Design review of the part built by this model. Coordinates are the model's own, in mm. A direction names the side the tool comes from. Give positions to 0.01 mm unless a question says otherwise; leave off trailing zeros. Write each loop counter-clockwise with the first axis right and the second up, starting at its lowest first coordinate (ties: lowest second). Pieces come first, ordered by that corner, then holes.
```python
from build123d import *

# Parameters (mm, degrees)
F0_W      = 38.1
F0_H      = 19.05
F1_DEPTH  = 50.8
F2_W      = 25.4
F2_H      = 19.05
F3_DEPTH  = 12.7
F5_DEPTH  = 31.75
F8_DEPTH  = 25.4
F10_DEPTH = 107.95
F11_W     = 38.1
F11_H     = 10.8646959405
F12_DEPTH = 50.8
F14_DEPTH = 25.4
F16_DEPTH = 25.4
F17_W     = 12.7
F17_H     = 10.8646959405
F18_DEPTH = 25.4
F6_W      = 2.6920993537
F6_H      = 9.7637060691
F19_DEPTH = 25.4
F20_DEPTH = 25.4
F21_W     = 11.8566676974
F21_H     = 11.0813332722
F22_DEPTH = 6.35
F23_W     = 4.0861964226
F23_H     = 3.3253813162
F23_W_2   = 3.8762353361
F23_H_2   = 3.7055220455
F23_W_3   = 3.8942359388
F23_H_3   = 4.0504299104
F24_DEPTH = 6.35
F26_DEPTH = 38.1
F28_DEPTH = 38.1
F30_DEPTH = 25.4


with BuildPart() as f1:
    # F0 (on Right) → F1 (new body)
    with BuildSketch(Plane.YZ):
        with Locations((42.7892319858, 20.3896959405)):
            Rectangle(F0_W, F0_H)
        Polygon((23.7392319858, 29.9146959405), (61.8392319858, 29.9146959405), (42.9846160114, 42.6146959405), align=None)
    extrude(amount=F1_DEPTH)

    # F2 (on face) → F3 (join)
    with BuildSketch(Plane.XZ.offset(-23.7392319858)):
        with Locations((25.4, 20.3896959405)):
            Rectangle(F2_W, F2_H)
    extrude(amount=F3_DEPTH)

    # F4 (on face) → F5 (join)
    with BuildSketch(Plane.XZ.offset(-11.0392319858)):
        Polygon((25.4, 44.1137275976), (12.7, 29.9146959405), (38.1, 29.9146959405), align=None)
    extrude(amount=-F5_DEPTH)

    # F7 (on Top) → F8 (join)
    with BuildSketch(Plane.XY):
        Polygon((0, 23.8369237632), (0, 62.1323101223), (-40.3469242156, 62.1323101223), (-40.3469242156, -46.306155622), (0, -46.306155622), align=None)
    extrude(amount=F8_DEPTH)

    # F9 (on face) → F10 (join)
    with BuildSketch(Plane.XZ.offset(46.306155622)):
        Polygon((-20.1734621078, 54.5123107731), (-40.3469242156, 25.4), (0, 25.4), align=None)
    extrude(amount=-F10_DEPTH)

    # F11 (on face) → F12 (join)
    with BuildSketch(Plane.YZ.offset(50.8)):
        with Locations((42.7892319858, 5.4323479703)):
            Rectangle(F11_W, F11_H)
    extrude(amount=-F12_DEPTH)

    # F13 (on face) → F14 (join)
    with BuildSketch(Plane.XZ.offset(-11.0392319858)):
        Polygon((37.7532355487, 11.0308341682), (12.6882037148, 11.0308341682), (12.2203705832, 0), (37.7532355487, 0), align=None)
    extrude(amount=F14_DEPTH)

    # F15 (on face) → F16 (join)
    with BuildSketch(Plane.XZ.offset(14.3607680142)):
        Polygon((37.7532355487, 0), (37.7532355487, 5.5154170841), (12.6882037148, 5.5154170841), (12.2203705832, 0), align=None)
    extrude(amount=F16_DEPTH)

    # F17 (on face) → F18 (join)
    with BuildSketch(Plane.YZ.offset(38.1)):
        with Locations((17.3892319858, 5.4323479703)):
            Rectangle(F17_W, F17_H)
    extrude(amount=-F18_DEPTH)

    # F6 (on face) → F19 (cut)
    with BuildSketch(Plane.XZ.offset(-11.0392319858)):
        with Locations((26.7460496768, 15.7465489751)):
            Rectangle(F6_W, F6_H)
    extrude(amount=-F19_DEPTH, mode=Mode.SUBTRACT)

    # F20 (add): a face of the model
    f20_faces = [f1.faces().sort_by_distance(p)[0] for p in [
        (0, 42.8272968204, 31.4509034),
    ]]
    extrude(f20_faces, amount=F20_DEPTH)

    # F21 (on face) → F22 (cut)
    with BuildSketch(Plane(origin=(-40.3469242156, 0, 0), x_dir=(0, -1, 0), z_dir=(-1, 0, 0))):
        with Locations((-41.2407740951, 15.2060096152)):
            Rectangle(F21_W, F21_H)
    extrude(amount=-F22_DEPTH, mode=Mode.SUBTRACT)

    # F23 (on face) → F24 (join)
    with BuildSketch(Plane(origin=(-33.9969242156, 0, 0), x_dir=(0, -1, 0), z_dir=(-1, 0, 0))):
        with Locations((-45.1260097325, 15.3784635477)):
            Rectangle(F23_W, F23_H)
        with Locations((-41.1447938532, 15.3784635477)):
            Rectangle(F23_W_2, F23_H)
        with Locations((-41.1447938532, 18.8939152285)):
            Rectangle(F23_W_2, F23_H_2)
        with Locations((-37.2595582157, 15.3784635477)):
            Rectangle(F23_W_3, F23_H)
        with Locations((-41.1447938532, 11.6905579343)):
            Rectangle(F23_W_2, F23_H_3)
    extrude(amount=F24_DEPTH)

    # F25 (on face) → F26 (join)
    with BuildSketch(Plane.XZ.offset(-23.7392319858)):
        Polygon((38.1, 29.9146959405), (50.8, 29.9146959405), (50.8, 63.7161359191), (0, 63.7161359191), (0, 29.9146959405), align=None)
    extrude(amount=-F26_DEPTH)

    # F27 (on face) → F28 (join)
    with BuildSketch(Plane.XZ.offset(-23.7392319858)):
        Polygon((25.4, 83.0065757036), (0, 63.7161359191), (50.8, 63.7161359191), align=None)
    extrude(amount=-F28_DEPTH)

    # F29 (on face) → F30 (cut)
    with BuildSketch(Plane.XZ.offset(-23.7392319858)):
        Polygon((23.3422555029, 74.4133889675), (10.8735319227, 63.7161359191), (32.519716375, 63.7161359191), align=None)
    extrude(amount=-F30_DEPTH, mode=Mode.SUBTRACT)


solid = f1.part
```
(1) Mouldability with a two-part tool opening along X and no side actions: class faces 1 (the face through (27, 24, 20.628)), 2 (the face through (21, 61.839, 42)), 3 (the face through (-33.997, 45, 19)) as pulls with the +X half, pulls with the -X half, needs draft (parallel to the pull), parting line crosses it, or undercut.
Resolved:
face 1: undercut
face 2: needs draft
face 3: pulls with the -X half
(2) Consider section D-D, the plane z = 70.5. Give the boundary of the cut face in (x, y).
Resolved:
outline: (8.93, 23.74) - (18.78, 23.74) - (18.78, 49.14) - (26.7, 49.14) - (26.7, 23.74) - (41.87, 23.74) - (41.87, 61.84) - (8.93, 61.84) - close
(3) Consider section B-B, the plane z = 46. Give the boundary of the cut face in (x, y).
Resolved:
outline: (-26.07, -46.31) - (-14.27, -46.31) - (-14.27, 61.64) - (-26.07, 61.64) - close; (0, 23.74) - (50.8, 23.74) - (50.8, 61.84) - (0, 61.84) - close
(4) Consider section C-C, the plane y = -38. Give the boundary of the cut face in (x, z).
Resolved:
outline: (-40.35, 0) - (0, 0) - (0, 25.4) - (-20.17, 54.51) - (-40.35, 25.4) - close; (12.22, 0) - (37.75, 0) - (37.75, 5.52) - (12.69, 5.52) - close
(5) Consider section A-A, the plane y = 1.5. Give the boundary of the cut face in (x, z).
Resolved:
outline: (-40.35, 0) - (0, 0) - (0, 25.4) - (-20.17, 54.51) - (-40.35, 25.4) - close; (12.22, 0) - (37.75, 0) - (37.75, 11.03) - (12.69, 11.03) - close
(6) To check wall thickness, follow L1, parallel to Z at x = -36, y = 45; L2, parallel to Y at x = 44.5, z = 52; L3, parallel to Z at x = 26.5, y = -10.5. State the ranges of each line that lie inside material, in increasing order.
Resolved:
L1: z = 0 to 9.67, 13.72 to 17.04, 20.75 to 31.67
L2: y = 23.74 to 61.84
L3: z = 0 to 11.03
(7) Tool access review of faces 4 (the face through (12.458, -1.483, 5.593)), 5 (the face through (17.195, 36.261, 69.14)), 6 (the face through (12.7, 17, 15)), 7 (the face through (-37, 43.083, 19)): name each direction out of +Z, -Z, +X, -X, +Y, -Y from which nothing blocks a thin tool from reaching the whole face with its end or side.
Resolved:
face 4: +Z, -Y
face 5: -Y
face 6: +Z, -Z
face 7: -X
(8) Clearance check with flat-ended pins moving along their axes: P1, Ø5.5, axis at x = 24.5, z = 7.5, coming from the -Y side; P2, Ø2, axis at x = 23.5, y = 3.5, coming from the +Z side; P3, Ø12.5, axis at y = -6, z = 18, coming from the +X side. State where each tip first meets the part, or that it passes through.
Resolved:
P1: stops at y = -39.76
P2: stops at z = 11.03
P3: stops at x = 0
